Source: CAD feature listing. Evaluate the final solid. Frame: model axes, mm. Give positions to 0.01 mm unless a question says otherwise; leave off trailing zeros. Answer as a JSON object with one key per item and string values. Group by question number.
Item 1: Section query A-A on z = 4. Give the number of separate pieces and of enclosed holes in the cut face, plus the area to 3 significant figures.
Item 2: Ray query, probe 1 along Y at (x, z) = (95, 1.9); probe 2 along Y at (x, z) = (163, 0.5); probe 3 along Y at (x, z) = (194, 4.85). Return the intervals inside material, ascending. Write a range as from..to.
Item 3: First-contact query: pin 1 Ø3 at (y, z) = (214.5, 2) entering from +X; pin 2 Ø2 at (x, z) = (84.5, 2) entering from +Y; pin 3 Ø3 at (y, z) = (254, 4) entering from +X; pin 4 Ø1.8 at (x, y) = (265, 215) entering from +Z. Flat tips, straight axial feed; report the tip coordinate or a pass-through.
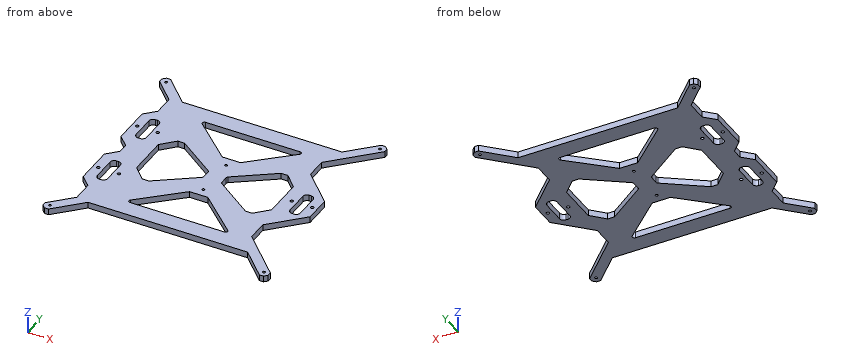
from build123d import *

# Parameters (mm, degrees)
FRAME_R             = 1.5
FRAME_R_2           = 1.25
BOSS_EXTRUDE1_DEPTH = 6


with BuildPart() as part:
    # FRAME → Boss-Extrude1 (new body)
    with BuildSketch(Plane.XY):
        Polygon((65, 325), (63, 325), (60, 322), (60, 320), (60, 318), (80, 298), (80, 278), (70, 268), (70, 230), (80, 220), (80, 210), (70, 200), (70, 162), (80, 152), (80, 132), (60, 112), (60, 108), (63, 105), (65, 105), (67, 105), (92, 130), (248, 130), (273, 105), (275, 105), (277, 105), (280, 108), (280, 112), (260, 132), (240, 152), (240, 172), (260, 192), (270, 202), (270, 228), (260, 238), (240, 258), (240, 278), (280, 318), (280, 321), (280, 322), (277, 325), (273, 325), (250, 302), (248, 300), (92, 300), (67, 325), align=None)
        with Locations((75, 250)):
            Circle(FRAME_R, mode=Mode.SUBTRACT)
        with Locations((95.037619408, 250)):
            Circle(FRAME_R, mode=Mode.SUBTRACT)
        with Locations((75, 180)):
            Circle(FRAME_R, mode=Mode.SUBTRACT)
        with Locations((95, 180)):
            Circle(FRAME_R, mode=Mode.SUBTRACT)
        with Locations((265, 215)):
            Circle(FRAME_R, mode=Mode.SUBTRACT)
        with Locations((245, 215)):
            Circle(FRAME_R, mode=Mode.SUBTRACT)
        with Locations((65.5, 319.5)):
            Circle(FRAME_R_2, mode=Mode.SUBTRACT)
        with Locations((274.5, 110.5)):
            Circle(FRAME_R_2, mode=Mode.SUBTRACT)
        with Locations((274.5, 319.5)):
            Circle(FRAME_R_2, mode=Mode.SUBTRACT)
        with Locations((65.5, 110.5)):
            Circle(FRAME_R_2, mode=Mode.SUBTRACT)
        with Locations((170.024675872, 194)):
            Circle(FRAME_R_2, mode=Mode.SUBTRACT)
        with Locations((170.024675872, 235)):
            Circle(FRAME_R_2, mode=Mode.SUBTRACT)
        with BuildLine():
            Line((161.216590497, 218.964796722), (161.216590497, 211.035203278))
            ThreePointArc((161.216590497, 211.035203278), (160.992764596, 210.115852653), (160.371384926, 209.402276511))
            Line((160.371384926, 209.402276511), (122.909474642, 182.909474642))
            Line((122.909474642, 182.909474642), (116.23015359, 182.909474642))
            Line((116.23015359, 182.909474642), (104.037619408, 195.501934511))
            Line((104.037619408, 195.501934511), (104.037619408, 234.498065489))
            Line((104.037619408, 234.498065489), (116.23015359, 247.090525358))
            Line((116.23015359, 247.090525358), (122.909474642, 247.090525358))
            Line((122.909474642, 247.090525358), (160.371384926, 220.597723489))
            ThreePointArc((160.371384926, 220.597723489), (160.992764596, 219.884147347), (161.216590497, 218.964796722))
        make_face(mode=Mode.SUBTRACT)
        with BuildLine():
            Line((122.471056888, 279.600410825), (161.114699893, 244.435797428))
            Line((161.114699893, 244.435797428), (178.934651851, 244.435797428))
            Line((178.934651851, 244.435797428), (217.578294856, 279.600410825))
            ThreePointArc((217.578294856, 279.600410825), (218.0975061, 281.801285282), (216.232236245, 283.079642455))
            Line((216.232236245, 283.079642455), (123.817115499, 283.079642455))
            ThreePointArc((123.817115499, 283.079642455), (121.951845644, 281.801285282), (122.471056888, 279.600410825))
        make_face(mode=Mode.SUBTRACT)
        with BuildLine():
            Line((217.139877102, 247.090525358), (179.677966818, 220.597723489))
            ThreePointArc((179.677966818, 220.597723489), (179.056587148, 219.884147347), (178.832761247, 218.964796722))
            Line((178.832761247, 218.964796722), (178.832761247, 211.035203278))
            ThreePointArc((178.832761247, 211.035203278), (179.056587148, 210.115852653), (179.677966818, 209.402276511))
            Line((179.677966818, 209.402276511), (217.139877102, 182.909474642))
            Line((217.139877102, 182.909474642), (223.819198154, 182.909474642))
            Line((223.819198154, 182.909474642), (236.011732336, 195.501934511))
            Line((236.011732336, 195.501934511), (236.011732336, 234.498065489))
            Line((236.011732336, 234.498065489), (223.819198154, 247.090525358))
            Line((223.819198154, 247.090525358), (217.139877102, 247.090525358))
        make_face(mode=Mode.SUBTRACT)
        with BuildLine():
            Line((217.578294856, 150.399589175), (178.934651851, 185.564202572))
            Line((178.934651851, 185.564202572), (161.114699893, 185.564202572))
            Line((161.114699893, 185.564202572), (122.471056888, 150.399589175))
            ThreePointArc((122.471056888, 150.399589175), (121.951845644, 148.198714718), (123.817115499, 146.920357545))
            Line((123.817115499, 146.920357545), (216.232236245, 146.920357545))
            ThreePointArc((216.232236245, 146.920357545), (218.0975061, 148.198714718), (217.578294856, 150.399589175))
        make_face(mode=Mode.SUBTRACT)
        with BuildLine():
            Line((80, 169), (80, 192))
            ThreePointArc((80, 192), (81.171572875, 194.828427125), (84, 196))
            Line((84, 196), (86, 196))
            ThreePointArc((86, 196), (88.828427125, 194.828427125), (90, 192))
            Line((90, 192), (90, 169))
            ThreePointArc((90, 169), (88.828427125, 166.171572875), (86, 165))
            Line((86, 165), (84, 165))
            ThreePointArc((84, 165), (81.171572875, 166.171572875), (80, 169))
        make_face(mode=Mode.SUBTRACT)
        with BuildLine():
            Line((80, 239.007036896), (80, 262.007036896))
            ThreePointArc((80, 262.007036896), (81.171572875, 264.835464021), (84, 266.007036896))
            Line((84, 266.007036896), (86, 266.007036896))
            ThreePointArc((86, 266.007036896), (88.828427125, 264.835464021), (90, 262.007036896))
            Line((90, 262.007036896), (90, 239.007036896))
            ThreePointArc((90, 239.007036896), (88.828427125, 236.178609771), (86, 235.007036896))
            Line((86, 235.007036896), (84, 235.007036896))
            ThreePointArc((84, 235.007036896), (81.171572875, 236.178609771), (80, 239.007036896))
        make_face(mode=Mode.SUBTRACT)
        with BuildLine():
            Line((250, 202.862876393), (250, 225.862876393))
            ThreePointArc((250, 225.862876393), (251.171572875, 228.691303518), (254, 229.862876393))
            Line((254, 229.862876393), (256, 229.862876393))
            ThreePointArc((256, 229.862876393), (258.828427125, 228.691303518), (260, 225.862876393))
            Line((260, 225.862876393), (260, 202.862876393))
            ThreePointArc((260, 202.862876393), (258.828427125, 200.034449268), (256, 198.862876393))
            Line((256, 198.862876393), (254, 198.862876393))
            ThreePointArc((254, 198.862876393), (251.171572875, 200.034449268), (250, 202.862876393))
        make_face(mode=Mode.SUBTRACT)
    extrude(amount=BOSS_EXTRUDE1_DEPTH)


solid = part.part
Worked answers:
{
 "1": {"separate pieces": "1", "enclosed holes": "19", "area": "21,100 mm^2"},
 "2": {"probe 1": "130..178.5, 181.5..248.5, 251.5..300", "probe 2": "130..146.92, 185.56..244.44, 283.08..300", "probe 3": "130..146.92, 171.86..199.27, 230.73..258.14, 283.08..300"},
 "3": {"pin 1": "x = 270", "pin 2": "y = 308.5", "pin 3": "x = 245.5", "pin 4": "through"}
}
